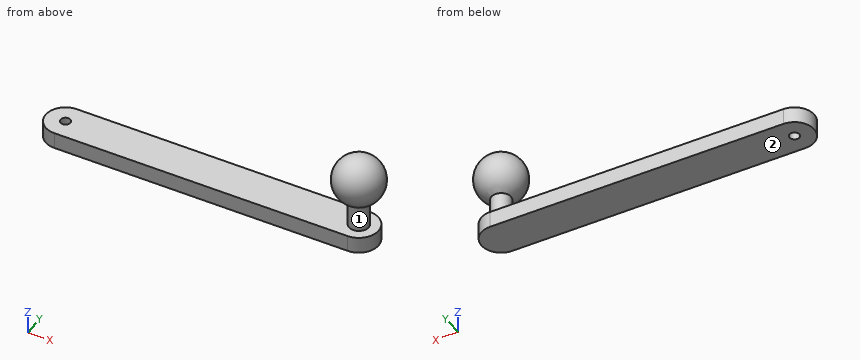
```python
from build123d import *

# Parameters (mm, degrees)
SKETCH1_R           = 1.5
BOSS_EXTRUDE1_DEPTH = 5
FILLET3_R           = 1
BOSS_EXTRUDE2_START = -5
SKETCH2_R           = 3
BOSS_EXTRUDE2_DEPTH = 20


with BuildPart() as part:
    # Sketch1 → Boss-Extrude1 (new body)
    with BuildSketch(Plane.XY):
        with BuildLine():
            ThreePointArc((0, 6), (-6, 0), (0, -6))
            Line((0, -6), (90, -6))
            ThreePointArc((90, -6), (96, 0), (90, 6))
            Line((90, 6), (0, 6))
        make_face()
        Circle(SKETCH1_R, mode=Mode.SUBTRACT)
        with Locations((90, 0)):
            Circle(SKETCH1_R, mode=Mode.SUBTRACT)
    extrude(amount=BOSS_EXTRUDE1_DEPTH)

    # Fillet3
    fillet3_edges = [part.edges().sort_by_distance(p)[0] for p in [
        (88.5, 0, 0),
    ]]
    fillet(fillet3_edges, radius=FILLET3_R)

    # Sketch2 → Boss-Extrude2 (add)
    with BuildSketch(Plane.XY.offset(5).offset(BOSS_EXTRUDE2_START)):
        with Locations((90, 0)):
            Circle(SKETCH2_R)
    extrude(amount=BOSS_EXTRUDE2_DEPTH)

    # Sketch3 → Revolve1 (revolve)
    with BuildSketch(Plane.XY.offset(20)):
        with BuildLine():
            Line((82.5, 0), (97.5, 0))
            ThreePointArc((97.5, 0), (90, 7.5), (82.5, 0))
        make_face()
    revolve(axis=Axis((90, 0, 20), (1, 0, 0)))


solid = part.part
```
Build history of the part. All positions in model axes, mm. Face numbers are marked on the shaded views. Give positions to 0.01 mm unless a question says otherwise; leave off trailing zeros. Loops run counter-clockwise (first coordinate to the right, second up) from the corner with the lowest first, then second, coordinate; pieces in that order, holes last.
1) Band-saw the part on B-B on x = 32.5. List the corners of the cut face in (y, z), then the cut area to 3 significant figures.
Values follow:
outline: (-6, 0) - (6, 0) - (6, 5) - (-6, 5) - close
area: 60.0 mm2
2) Band-saw the part on D-D on z = 21.75. List the corners of the cut face in (x, y), then the cut area to 3 significant figures.
Values follow:
outline: circle Ø14.59 at (90, 0)
area: 167 mm2
3) Probe line 1 along Z through (x, y) = (25.5, -1.5); line 2 along X through (y, z) = (-3.75, 14.25); line 3 along Y through (x, z) = (32.5, 4.5). List the from-to ranges inside material, lowest first.
Values follow:
line 1: z = 0 to 5
line 2: x = 86.98 to 93.02
line 3: y = -6 to 6
4) Band-saw the part on A-A on y = 0. List the corners of the cut face in (x, z), then the cut area to 3 significant figures.
Values follow:
outline: (-6, 0) - (-1.5, 0) - (-1.5, 5) - (-6, 5) - close; (1.5, 0) - (96, 0) - (96, 5) - (93, 5) - (93, 13.13) arc R7.5 ccw (long way) to (87, 13.13) - (87, 5) - (1.5, 5) - close
area: 718 mm2
5) Band-saw the part on C-C on z = 17.5. List the corners of the cut face in (x, y), then the cut area to 3 significant figures.
Values follow:
outline: circle Ø14.14 at (90, 0)
area: 157 mm2
6) Drop flat-ended pins along their axis: P1, Ø1.5, axis at y = 2, z = 20, coming from the +X side; P2, Ø5, axis at y = -4, z = 18, coming from the +X side; P3, Ø4, axis at x = 52, z = 2, coming from the -Y side. Give the stop position or say it passes through.
Values follow:
P1: stops at x = 97.4
P2: stops at x = 97.24
P3: stops at y = -6
7) Two-plate mould, pull along Z, no slides. Class the marked faces 1 and 2: released by +Z, released by -Z, zero draft, split by the parting line, or undercut.
Values follow:
face 1: undercut
face 2: released by -Z
